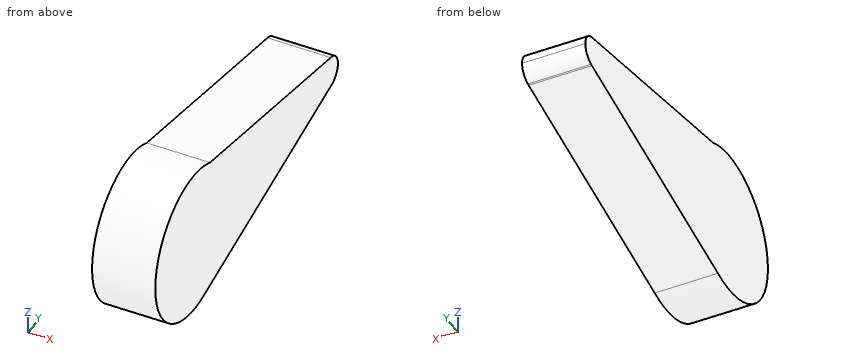
from build123d import *

# Parameters (mm, degrees)
F1_DEPTH = 25


with BuildPart() as f1:
    # F0 (on Right) → F1 (new body)
    with BuildSketch(Plane.YZ):
        with BuildLine():
            ThreePointArc((5.81453, -31.705164), (20.904065, -20.916165), (26.680938, -3.288791))
            ThreePointArc((26.680938, -3.288791), (21.999843, 12.73976), (9.428084, 23.729661))
            ThreePointArc((9.428084, 23.729661), (-32.820494, -1.351527), (5.81453, -31.705164))
        make_face()
        with BuildLine():
            ThreePointArc((9.428084, 23.729661), (21.999843, 12.73976), (26.680938, -3.288791))
            ThreePointArc((26.680938, -3.288791), (20.904065, -20.916165), (5.81453, -31.705164))
            Line((5.81453, -31.705164), (103.305496, -6.28672))
            ThreePointArc((103.305496, -6.28672), (95.581705, -0.235054), (102.842035, 6.365493))
            Line((102.842035, 6.365493), (9.428084, 23.729661))
        make_face()
        with BuildLine():
            ThreePointArc((108.419674, 0), (106.827989, 4.231712), (102.842035, 6.365493))
            ThreePointArc((102.842035, 6.365493), (95.581705, -0.235054), (103.305496, -6.28672))
            Line((103.305496, -6.28672), (103.92752, -6.124542))
            ThreePointArc((103.92752, -6.124542), (107.176242, -3.797679), (108.419674, 0))
        make_face()
    extrude(amount=F1_DEPTH)


solid = f1.part
Check sheet for the modelled part. Datum: model origin and axes. Units: mm. Give positions to 0.01 mm unless a question says otherwise; leave off trailing zeros. Loops run counter-clockwise (first coordinate to the right, second up) from the corner with the lowest first, then second, coordinate; pieces in that order, holes last. Notation, with made-up numbers: M 11,-11 L 55,-11 A30 cw 55,23 Z; hole C 71,-26.5 d7. An arc over 180 degrees is marked long. Return JSON: item names as keys, results as strings. Group by question number.
1. Go/stop test with flat-tipped pins: pin 1 (4 mm diameter, centred on x = 16.5, y = 60.5, fed in from +Z); pin 2 (2 mm diameter, centred on x = 16, y = 2.5, fed in from +Z); pin 3 (1 mm diameter, centred on x = 8, y = 13, fed in from +Z). Record where each tip stops, or that it passes through.
2. Cross-section at C-C on y = 47. Record the boundary of the cut face in (x, z), plus the area to 3 significant figures.
3. Cross-section at B-B on z = -18. Record the boundary of the cut face in (x, y), plus the area to 3 significant figures.
4. Thickness scan on L1, parallel to Z at x = 8.25, y = 85.5; L2, parallel to Y at x = 16.75, z = 4; L3, parallel to Z at x = 20.25, y = 13.5. Record the ranges inside material, lowest first.
5. Cross-section at A-A on x = 21.75. Record the boundary of the cut face in (y, z).
Return value:
{
 "1": {"pin 1": "z = 14.61", "pin 2": "z = 26.14", "pin 3": "z = 23.16"},
 "2": {"outline": "M 0,-20.97 L 25,-20.97 L 25,16.75 L 0,16.75 Z", "area": "943 mm^2"},
 "3": {"outline": "M 0,-29 L 25,-29 L 25,58.38 L 0,58.38 Z", "area": "2,180 mm^2"},
 "4": {"L1": "-10.93 to 9.59", "L2": "-31.98 to 107.02", "L3": "-29.7 to 22.97"},
 "5": {"outline": "M 5.81,-31.71 L 103.31,-6.29 L 103.93,-6.12 A6.42 ccw 108.42,0 A6.42 ccw 102.84,6.37 L 9.43,23.73 A29.78 ccw long Z"}
}
